from build123d import *

# Parameters (mm, degrees)
BOSS_EXTRUDE1_DEPTH = 4.78
SKETCH2_R           = 4.05
CUT_EXTRUDE1_DEPTH  = 4.78
CIRPATTERN1_COUNT   = 6
CIRPATTERN2_COUNT   = 4


with BuildPart() as part:
    # Sketch1 → Boss-Extrude1 (new body)
    with BuildSketch(Plane(origin=(0, 0, 0), x_dir=(1, 0, 0), z_dir=(0, 1, 0))):
        Polygon((160, 0), (80, 138.564064606), (-80, 138.564064606), (-160, 0), (-80, -138.564064606), (80, -138.564064606), align=None)
    extrude(amount=BOSS_EXTRUDE1_DEPTH)

    # Sketch2 → Cut-Extrude1 (cut)
    with BuildSketch(Plane(origin=(0, 4.78, 0), x_dir=(1, 0, 0), z_dir=(0, 1, 0))):
        with Locations(Location((0, -123.564064606, 0), (0, 0, 270))):
            Circle(SKETCH2_R)
        with Locations(Location((0, -108.564064606, 0), (0, 0, 270))):
            Circle(SKETCH2_R)
    cut_extrude1 = extrude(amount=-CUT_EXTRUDE1_DEPTH, mode=Mode.SUBTRACT)

    # CirPattern1: Cut-Extrude1 ×6 about axis
    cirpattern1_axis = Axis((0, 0, -0.180123057), (0, 1, 0))
    for i in range(1, CIRPATTERN1_COUNT):
        add(cut_extrude1.rotate(cirpattern1_axis, i * 360 / CIRPATTERN1_COUNT), mode=Mode.SUBTRACT)

    # CirPattern2: Cut-Extrude1 ×4 about axis
    cirpattern2_axis = Axis((0, 0, 0.001690344), (0, 1, 0))
    for i in range(1, CIRPATTERN2_COUNT):
        add(cut_extrude1.rotate(cirpattern2_axis, i * 360 / CIRPATTERN2_COUNT), mode=Mode.SUBTRACT)


solid = part.part
Verification items for the finished model (mm, model axes). Round coordinates to 2 decimals unless told otherwise and drop trailing zeros. Order: outer loops, then holes, each group sorted by start corner. A loop starts at its lowest first (then second) coordinate and runs counter-clockwise, first axis right, second up. Notation, with made-up numbers: (48, 80.5) -> (88, 80.5) arc R34 cw to (88, 114.5) -> close; hole circle Ø1 at (-2, 9.25). An arc over 180 degrees is marked (long way). Put each result on its own line as item: value.
1) Section check D-D (x = -131.5). Record the cut outline in (y, z).
Final values:
outline: (0, -49.36) -> (4.78, -49.36) -> (4.78, 49.36) -> (0, 49.36) -> close
2) Section check B-B (y = 1.4). Give the number of separate pieces and of enclosed holes in the cut face, then the cut area to 3 significant figures.
Final values:
separate pieces: 1
enclosed holes: 16
area: 65,700 mm^2
3) Material ranges on line 1 (Z direction, x = 0.5, y = 4.55); line 2 (Z direction, x = -97, y = 2.6); line 3 (X direction, y = 3.7, z = -96), recorded low to high.
Final values:
line 1: z = -138.56 to -127.94, -119.54 to -112.94, -104.54 to 104.55, 112.58 to 119.55, 127.58 to 138.56
line 2: z = -109.12 to -57.45, -51.65 to 51.29, 57.09 to 109.12
line 3: x = -104.57 to 104.57
4) Section check C-C (z = -32). Record the cut outline in (x, y), then the cut area to 3 significant figures.
Final values:
outline: (-141.52, 0) -> (141.52, 0) -> (141.52, 4.78) -> (-141.52, 4.78) -> close
area: 1,350 mm^2
5) Mould release check, pull along X, two halves, no side actions. Record for faces 1 (the cylindrical face through (-112.304, 2.423, -1.549)), 2 (the cylindrical face through (-90.22, 2.42, 55.07)), 3 (the flat face through (119.44, 2.36, 70.25)), 4 (the flat face through (-119.44, 2.36, -70.25)): +X half, -X half, draft (parallel to the pull), parting line (faces both ways), or undercut.
Final values:
face 1: undercut
face 2: undercut
face 3: +X half
face 4: -X half
6) Depth check by flat-ended pin: pin 1 (13 mm diameter, centred on x = -107.17, z = 61.69, fed in from +Y). Enter the tip coordinate at first touch or a pass-through.
Final values:
pin 1: stops at y = 4.78
7) Section check A-A (x = 0). Record the cut outline in (y, z), then the cut area to 3 significant figures.
Final values:
outline: (0, -138.56) -> (4.78, -138.56) -> (4.78, -127.97) -> (0, -127.97) -> close; (0, -119.51) -> (4.78, -119.51) -> (4.78, -112.97) -> (0, -112.97) -> close; (0, -104.51) -> (4.78, -104.51) -> (4.78, 104.51) -> (0, 104.51) -> close; (0, 112.61) -> (4.78, 112.61) -> (4.78, 119.51) -> (0, 119.51) -> close; (0, 127.61) -> (4.78, 127.61) -> (4.78, 138.56) -> (0, 138.56) -> close
area: 1,170 mm^2
